from build123d import *

# Parameters (mm, degrees)
SKETCH1_W           = 32
SKETCH1_H           = 32
BOSS_EXTRUDE2_DEPTH = 20
SKETCH2_R           = 14.5
BOSS_EXTRUDE3_DEPTH = 46
SKETCH3_R           = 7
BOSS_EXTRUDE4_DEPTH = 6
SKETCH6_R           = 6
BOSS_EXTRUDE5_DEPTH = 1.2
SKETCH7_R           = 1.5
BOSS_EXTRUDE6_DEPTH = 10
CUT_EXTRUDE5_DEPTH  = 20


with BuildPart() as part:
    # Sketch1 → Boss-Extrude2 (new body)
    with BuildSketch(Plane(origin=(0, 0, 0), x_dir=(0, 0, -1), z_dir=(1, 0, 0))):
        Rectangle(SKETCH1_W, SKETCH1_H)
    extrude(amount=BOSS_EXTRUDE2_DEPTH)

    # Sketch2 → Boss-Extrude3 (add)
    with BuildSketch(Plane.ZY):
        Circle(SKETCH2_R)
    extrude(amount=BOSS_EXTRUDE3_DEPTH)

    # Sketch3 → Boss-Extrude4 (add)
    with BuildSketch(Plane(origin=(20, 0, 0), x_dir=(0, 0, -1), z_dir=(1, 0, 0))):
        with Locations(Location((0, 0, 0), (0, 0, 180))):
            Circle(SKETCH3_R)
    extrude(amount=BOSS_EXTRUDE4_DEPTH)

    # Sketch6 → Boss-Extrude5 (add)
    with BuildSketch(Plane(origin=(26, 0, 0), x_dir=(0, 0, -1), z_dir=(1, 0, 0))):
        Circle(SKETCH6_R)
    extrude(amount=BOSS_EXTRUDE5_DEPTH)

    # Sketch7 → Boss-Extrude6 (add)
    with BuildSketch(Plane(origin=(27.2, 0, 0), x_dir=(0, 0, -1), z_dir=(1, 0, 0))):
        Circle(SKETCH7_R)
    extrude(amount=BOSS_EXTRUDE6_DEPTH)

    # Sketch8 → Cut-Extrude5 (cut)
    with BuildSketch(Plane(origin=(20, 0, 0), x_dir=(0, 0, -1), z_dir=(1, 0, 0))):
        with BuildLine():
            ThreePointArc((-14.5, -13), (-14.060660172, -14.060660172), (-13, -14.5))
            Line((-13, -14.5), (-13, -13))
            Line((-13, -13), (-14.5, -13))
        make_face()
        with BuildLine():
            Line((-13, -13), (-13, -14.5))
            ThreePointArc((-13, -14.5), (-11.939339828, -14.060660172), (-11.5, -13))
            ThreePointArc((-11.5, -13), (-13, -11.5), (-14.5, -13))
            Line((-14.5, -13), (-13, -13))
        make_face()
        with BuildLine():
            ThreePointArc((14.5, -13), (11.939339828, -11.939339828), (13, -14.5))
            Line((13, -14.5), (13, -13))
            Line((13, -13), (14.5, -13))
        make_face()
        with BuildLine():
            Line((13, -13), (13, -14.5))
            ThreePointArc((13, -14.5), (14.060660172, -14.060660172), (14.5, -13))
            Line((14.5, -13), (13, -13))
        make_face()
        with BuildLine():
            ThreePointArc((14.5, 13), (14.060660172, 14.060660172), (13, 14.5))
            Line((13, 14.5), (13, 13))
            Line((13, 13), (14.5, 13))
        make_face()
        with BuildLine():
            Line((13, 13), (13, 14.5))
            ThreePointArc((13, 14.5), (11.939339828, 11.939339828), (14.5, 13))
            Line((14.5, 13), (13, 13))
        make_face()
        with BuildLine():
            ThreePointArc((-11.5, 13), (-11.939339828, 14.060660172), (-13, 14.5))
            Line((-13, 14.5), (-13, 13))
            Line((-13, 13), (-14.5, 13))
            ThreePointArc((-14.5, 13), (-13, 11.5), (-11.5, 13))
        make_face()
        with BuildLine():
            Line((-13, 13), (-13, 14.5))
            ThreePointArc((-13, 14.5), (-14.060660172, 14.060660172), (-14.5, 13))
            Line((-14.5, 13), (-13, 13))
        make_face()
    extrude(amount=-CUT_EXTRUDE5_DEPTH, mode=Mode.SUBTRACT)


solid = part.part
Geometry check sheet. Reference: the model listing, model coordinates, mm. A direction names the side the tool comes from. Give positions to 0.01 mm unless a question says otherwise; leave off trailing zeros. Write each loop counter-clockwise with the first axis right and the second up, starting at its lowest first coordinate (ties: lowest second). Pieces come first, ordered by that corner, then holes. Notation, with made-up numbers: (48, -3.5) - (77, -3.5) arc R30 cw to (77, 27.5) - close; hole circle Ø1 at (-0.5, -35). An arc over 180 degrees is marked (long way). Put each result on its own line as item: value.
1. Sectioned sample at D-D, the plane z = -10. Enter the section's corners in (x, y).
Ans:
outline: (-46, -10.5) - (0, -10.5) - (0, -16) - (20, -16) - (20, 16) - (0, 16) - (0, 10.5) - (-46, 10.5) - close
2. Thickness scan on line 1 (Z direction, x = 12, y = 13); line 2 (Z direction, x = 19, y = 14). Record the ranges inside material, lowest first.
Ans:
line 1: z = -16 to -14.5, -11.5 to 11.5, 14.5 to 16
line 2: z = -16 to -14.12, -11.88 to 11.88, 14.12 to 16
3. Set-up check for faces 1 (the flat face through (0, 3.6, 14.3)), 2 (the flat face through (20, 0.2, 7.3)), 3 (the flat face through (10, 0, 16)): record each of +Z, -Z, +X, -X, +Y, -Y from which the full face is reachable in a straight line by a thin tool's end or side.
Ans:
face 1: -X
face 2: +X
face 3: +Z, +X, -X, +Y, -Y
4. Go/stop test with flat-tipped pins: pin 1 (5 mm diameter, centred on y = 13, z = -13, fed in from +X); pin 2 (16 mm diameter, centred on y = -5, z = 4.5, fed in from +X); pin 3 (2.5 mm diameter, centred on y = -13, z = -13, fed in from +X); pin 4 (1 mm diameter, centred on x = -34.5, y = 8.5, fed in from +Z). Record where each tip stops, or that it passes through.
Ans:
pin 1: stops at x = 20
pin 2: stops at x = 37.2
pin 3: passes through
pin 4: stops at z = 12.09
5. Sectioned sample at B-B, the plane x = -5. Enter the section's corners in (y, z), plus the area to 3 significant figures.
Ans:
outline: circle Ø29 at (0, 0)
area: 661 mm²
6. Sectioned sample at C-C, the plane y = -3. Enter the section's corners in (x, z), plus the area to 3 significant figures.
Ans:
outline: (-46, -14.19) - (0, -14.19) - (0, -16) - (20, -16) - (20, -6.32) - (26, -6.32) - (26, -5.2) - (27.2, -5.2) - (27.2, 5.2) - (26, 5.2) - (26, 6.32) - (20, 6.32) - (20, 16) - (0, 16) - (0, 14.19) - (-46, 14.19) - close
area: 2,030 mm²
7. Sectioned sample at A-A, the plane z = 0. Enter the section's corners in (x, y), plus the area to 3 significant figures.
Ans:
outline: (-46, -14.5) - (0, -14.5) - (0, -16) - (20, -16) - (20, -7) - (26, -7) - (26, -6) - (27.2, -6) - (27.2, -1.5) - (37.2, -1.5) - (37.2, 1.5) - (27.2, 1.5) - (27.2, 6) - (26, 6) - (26, 7) - (20, 7) - (20, 16) - (0, 16) - (0, 14.5) - (-46, 14.5) - close
area: 2,100 mm²
